from build123d import *

# Parameters (mm, degrees)
BOSS_EXTRUDE1_DEPTH = 3
SKETCH2_R           = 1.25
CUT_EXTRUDE1_DEPTH  = 3
FILLET1_R           = 3


with BuildPart() as part:
    # Sketch1 → Boss-Extrude1 (new body)
    with BuildSketch(Plane.XY):
        Polygon((-56.024750416, -23.482321131), (-9.384750416, -23.482321131), (-5.192883407, 0.290938026), (2.685578617, -1.098247395), (-2.671953367, -31.482321131), (-48.024750416, -31.482321131), align=None)
    extrude(amount=BOSS_EXTRUDE1_DEPTH)

    # Sketch2 → Cut-Extrude1 (cut)
    with BuildSketch(Plane.XY.offset(3)):
        with Locations((-6.028351891, -27.482321131)):
            Circle(SKETCH2_R)
        Polygon((-56.024750416, -23.482321131), (-41.024750416, -23.482321131), (-41.024750416, -25.482321131), (-54.024750416, -25.482321131), align=None)
        with BuildLine():
            Line((-3.251155147, -2.590007585), (-6.203174167, -19.331739386))
            ThreePointArc((-6.203174167, -19.331739386), (-4.915458342, -21.170788176), (-3.076409552, -19.88307235))
            Line((-3.076409552, -19.88307235), (-0.124390531, -3.141340549))
            ThreePointArc((-0.124390531, -3.141340549), (-1.412106357, -1.302291759), (-3.251155147, -2.590007585))
        make_face()
    extrude(amount=-CUT_EXTRUDE1_DEPTH, mode=Mode.SUBTRACT)

    # Fillet1
    fillet1_edges = [part.edges().sort_by_distance(p)[0] for p in [
        (-5.192883407, 0.290938026, 1.5),
        (2.685578617, -1.098247395, 1.5),
        (-2.671953367, -31.482321131, 1.5),
    ]]
    fillet(fillet1_edges, radius=FILLET1_R)


solid = part.part
Work out the finished part from the listing and answer in its coordinate system (mm). A direction names the side the tool comes from. Round coordinates to 2 decimals unless told otherwise and drop trailing zeros. Write each loop counter-clockwise with the first axis right and the second up, starting at its lowest first coordinate (ties: lowest second). Pieces come first, ordered by that corner, then holes.
1) The mould has two halves that part along Y. Classify faces 4 (the flat face through (-47, -25.482, 2)), 5 (the cylindrical face through (-3.283, -30.799, 1.521)), 6 (the cylindrical face through (-4.95, -21.164, 1.521)): pulls with the +Y half, pulls with the -Y half, needs draft (parallel to the pull), parting line crosses it, or undercut.
2) A cutting plane is placed at C-C (x = -46.5). Give the vertices of the cut face in (y, z), plus the area to 3 significant figures.
3) A cutting plane is placed at A-A (y = -18). Give the vertices of the cut face in (x, z).
4) A cutting plane is placed at D-D (x = -37). Give the vertices of the cut face in (y, z), plus the area to 3 significant figures.
5) A tool of negligible diameter and unlimited length cuts with its end or side. For faces 1 (the flat face through (-41.025, -24, 2)), 2 (the flat face through (-4.7, -10.8, 1.5)), 3 (the flat face through (-20, -24, 3)), from which of +Z, -Z, +X, -X, +Y, -Y can it reach the whole face along a straight path? Write none if from no direction.
6) Straight lines are drawn through the part: line 1 (Y direction, x = -44, z = 1); line 2 (X direction, y = -11.5, z = 0.65); line 3 (X direction, y = -26.5, z = 1.45). For each, find the intervals that lie inside material, in ascending order.
7) A cutting plane is placed at B-B (z = 0.65). Give the number of separate pieces and of enclosed holes in the cut face, plus the area to 3 significant figures.
8) Given pin 1 Ø1.5 at (y, z) = (-19.5, 0.5) entering from +X; pin 2 Ø1.5 at (x, z) = (-47.5, 2) entering from +Y; pin 3 Ø8 at (x, y) = (-12.5, -3.5) entering from -Z; pin 4 Ø1.5 at (x, z) = (-28.5, 1) entering from +Y, each flat-ended and moving along its own axis, determine where each tip first touches the part or whether it passes through.
Completed:
1. face 4: pulls with the +Y half
1. face 5: pulls with the -Y half
1. face 6: undercut
2. outline: (-31.48, 0) - (-25.48, 0) - (-25.48, 3) - (-31.48, 3) - close
2. area: 18.0 mm2
3. outline: (-8.42, 0) - (-5.97, 0) - (-5.97, 3) - (-8.42, 3) - close; (-2.74, 0) - (-0.29, 0) - (-0.29, 3) - (-2.74, 3) - close
4. outline: (-31.48, 0) - (-23.48, 0) - (-23.48, 3) - (-31.48, 3) - close
4. area: 24.0 mm2
5. face 1: +Z, -Z, -X, +Y
5. face 2: +Z, -Z
5. face 3: +Z, +X, -X, +Y, -Y
6. line 1: y = -31.48 to -25.48
6. line 2: x = -7.27 to -4.82, -1.6 to 0.85
6. line 3: x = -53.01 to -6.8, -5.26 to -1.79
7. separate pieces: 1
7. enclosed holes: 2
7. area: 488 mm2
8. pin 1: stops at x = -0.43
8. pin 2: stops at y = -25.48
8. pin 3: passes through
8. pin 4: stops at y = -23.48
